from build123d import *

# Parameters (mm, degrees)
F0_W     = 14.3263228238
F0_H     = 64.4684862345
F0_W_2   = 16.372948885
F0_W_3   = 15.3496470302
F0_W_4   = 24.5594233274
F0_H_2   = 19.4428749382
F1_DEPTH = 50.8
F2_W     = 8.8241882622
F2_H     = 89.1295920778
F3_DEPTH = 38.1
F5_D     = 33.02


with BuildPart() as f1:
    # F0 (on Right) → F1 (new body)
    with BuildSketch(Plane.YZ):
        with Locations((69.4126244634, -3.0189463869)):
            Rectangle(F0_W, F0_H)
        with Locations((54.0629886091, -3.0189463869)):
            Rectangle(F0_W_2, F0_H)
        with Locations((38.2016906515, -3.0189463869)):
            Rectangle(F0_W_3, F0_H)
        Polygon((30.5268671364, -35.2531895041), (30.5268671364, 29.2152967304), (0, 29.2152967304), (0, -15.8103145659), (-52.3611754179, -15.8103145659), (-52.3611754179, -35.2531895041), align=None)
        Polygon((0, -15.8103145659), (0, 29.2152967304), (-76.9205987453, -15.8103145659), (-52.3611754179, -15.8103145659), align=None)
        with Locations((-64.6408870816, -25.531752035)):
            Rectangle(F0_W_4, F0_H_2)
    extrude(amount=F1_DEPTH)

    # F2 (on face) → F3 (join)
    with BuildSketch(Plane(origin=(0, -12.7370466018, 21.7596435151), x_dir=(1, 0, 0), z_dir=(0, -0.5051701713, 0.8630197553))):
        with Locations((25.8237272501, -29.8060995855)):
            Rectangle(F2_W, F2_H)
    extrude(amount=F3_DEPTH)

    # F5 (through all)
    with Locations(Plane.XY.offset(29.2152967304)):
        with Locations((25.8237272501, 38.6297218502)):
            Hole(F5_D / 2)


solid = f1.part
Design review of the part built by this model. Coordinates are the model's own, in mm. A direction names the side the tool comes from. Give positions to 0.01 mm unless a question says otherwise; leave off trailing zeros. Order: outer loops, then holes, each group sorted by start corner. A loop starts at its lowest first (then second) coordinate and runs counter-clockwise, first axis right, second up.
1. Mouldability with a two-part tool opening along Y and no side actions: class faces 1 (the flat face through (25, -76.921, -26)), 2 (the flat face through (8, 39, 29.215)), 3 (the cylindrical face through (27.97, 55, -3.47)), 4 (the flat face through (25.76, -9.49, 45.43)) as +Y half, -Y half, draft (parallel to the pull), parting line (faces both ways), or undercut.
Solution:
face 1: -Y half
face 2: draft
face 3: undercut
face 4: +Y half
2. Tool access review of faces 5 (the flat face through (30.236, -48, 23)), 6 (the flat face through (21.412, -48, 23)), 7 (the flat face through (0, 16, -10)): name each direction out of +Z, -Z, +X, -X, +Y, -Y from which nothing blocks a thin tool from reaching the whole face with its end or side.
Solution:
face 5: +Z, +X, -Y
face 6: +Z, -X, -Y
face 7: +Z, -Z, -X, +Y, -Y
3. For pin 1 Ø15.5 at (x, z) = (36.5, -23.5) entering from -Y; pin 2 Ø10 at (x, z) = (28.5, 48.5) entering from +Y; pin 3 Ø12 at (x, z) = (39, 22.5) entering from -Y, all flat-tipped, find the tip position at first contact; note any pin that passes through.
Solution:
pin 1: stops at y = -76.92
pin 2: stops at y = -8.36
pin 3: stops at y = -21.72
4. Add section D-D, the plane x = 6. State the section outline as (y, z) points, then the cut area to 3 significant figures.
Solution:
outline: (-76.92, -35.25) - (76.58, -35.25) - (76.58, 29.22) - (0, 29.22) - (-76.92, -15.81) - close
area: 8,160 mm2
5. Add section C-C, the plane y = 29. State the section outline as (x, z) points.
Solution:
outline: (0, -35.25) - (12.41, -35.25) - (12.41, 29.22) - (0, 29.22) - close; (39.23, -35.25) - (50.8, -35.25) - (50.8, 29.22) - (39.23, 29.22) - close
6. To check wall thickness, follow L1, parallel to Z at x = 27, y = 70.5; L2, parallel to Y at x = 12, z = -3.5; L3, parallel to Y at x = 25.5, z = 24. State the ranges of each line that lie inside material, in increasing order.
Solution:
L1: z = -35.25 to 29.22
L2: y = -55.89 to 29.6, 47.66 to 76.58
L3: y = -84.33 to 22.12, 55.14 to 76.58
7. Add section A-A, the plane x = 18. State the section outline as (y, z) points, then the cut area to 3 significant figures.
Solution:
outline: (-76.92, -35.25) - (24.09, -35.25) - (24.09, 29.22) - (0, 29.22) - (-76.92, -15.81) - close; (53.17, -35.25) - (76.58, -35.25) - (76.58, 29.22) - (53.17, 29.22) - close
area: 6,290 mm2
8. Add section B-B, the plane z = 27.5. State the section outline as (x, y) points, then the cut area to 3 significant figures.
Solution:
outline: (0, -2.93) - (21.41, -2.93) - (21.41, -78.35) - (30.24, -78.35) - (30.24, -2.93) - (50.8, -2.93) - (50.8, 76.58) - (0, 76.58) - close; hole circle Ø33.02 at (25.82, 38.63)
area: 3,850 mm2
